from build123d import *

# Parameters (mm, degrees)
SKETCH1_W                                            = 380
SKETCH1_H                                            = 68
BOSS_EXTRUDE1_DEPTH                                  = 25
SKETCH2_R                                            = 28.5
CUT_EXTRUDE1_DEPTH                                   = 195.630419
CUT_EXTRUDE2_DEPTH                                   = 195.630419
CUT_EXTRUDE2_DEPTH_BACK                              = 195.630419
SKETCH4_R                                            = 9.55
CHAMFER1_SIZE                                        = 0.5
FILLET1_R                                            = 12
M8_CLEARANCE_HOLE1_D                                 = 9
CHAMFER2_SIZE                                        = 0.5
CHAMFER3_SIZE                                        = 0.5
M6X1_0_TAPPED_HOLE1_D                                = 5
SKETCH13_R                                           = 13.411040831
SKETCH13_R_2                                         = 14.724493856
BOSS_EXTRUDE3_DEPTH                                  = 8
CSK_FOR_5_16_FLAT_HEAD_SOCKET_CAP_SCREW1_D           = 8.4328
CSK_FOR_5_16_FLAT_HEAD_SOCKET_CAP_SCREW1_CSINK_D     = 18.4009792
CSK_FOR_5_16_FLAT_HEAD_SOCKET_CAP_SCREW1_CSINK_ANGLE = 82


with BuildPart() as part:
    # Sketch1 → Boss-Extrude1 (new body)
    with BuildSketch(Plane(origin=(0, 0, 0), x_dir=(1, 0, 0), z_dir=(0, 1, 0))):
        Rectangle(SKETCH1_W, SKETCH1_H)
    extrude(amount=BOSS_EXTRUDE1_DEPTH)

    # Sketch2 → Cut-Extrude1 (cut, through all)
    with BuildSketch(Plane(origin=(0, 25, 0), x_dir=(1, 0, 0), z_dir=(0, 1, 0))):
        with Locations(Location((-134, 0, 0), (0, 0, 270))):
            Circle(SKETCH2_R)
        with Locations(Location((134, 0, 0), (0, 0, 270))):
            Circle(SKETCH2_R)
    extrude(amount=-CUT_EXTRUDE1_DEPTH, mode=Mode.SUBTRACT)

    # Sketch4 → Cut-Extrude2 (cut, two sides: drawn at the far end of the back side and taken through both)
    with BuildSketch(Plane(origin=(0, 25, 0), x_dir=(1, 0, 0), z_dir=(0, 1, 0)).offset(-CUT_EXTRUDE2_DEPTH_BACK)):
        with Locations(Location((-46, 0, 0), (0, 0, 270))):
            Circle(SKETCH4_R)
        with Locations(Location((46, 0, 0), (0, 0, 270))):
            Circle(SKETCH4_R)
    extrude(amount=CUT_EXTRUDE2_DEPTH + CUT_EXTRUDE2_DEPTH_BACK, mode=Mode.SUBTRACT)

    # Chamfer1
    chamfer1_edges = [part.edges().sort_by_distance(p)[0] for p in [
        (-134, 0, -28.5),
        (-134, 25, -28.5),
        (134, 0, -28.5),
        (134, 25, -28.5),
        (-46, 0, -9.55),
        (-46, 25, -9.55),
        (46, 0, -9.55),
        (46, 25, -9.55),
    ]]
    chamfer(chamfer1_edges, length=CHAMFER1_SIZE)

    # Fillet1
    fillet1_edges = [part.edges().sort_by_distance(p)[0] for p in [
        (190, 12.5, 34),
        (-190, 12.5, 34),
        (-190, 12.5, -34),
        (190, 12.5, -34),
    ]]
    fillet(fillet1_edges, radius=FILLET1_R)

    # M8 Clearance Hole1 (through all)
    with Locations(Plane.XZ):
        with Locations((-178, -22), (-178, 22), (178, -22), (178, 22)):
            Hole(M8_CLEARANCE_HOLE1_D / 2)

    # Chamfer2
    chamfer2_edges = [part.edges().sort_by_distance(p)[0] for p in [
        (190, 0, 0),
        (0, 0, 34),
        (-190, 0, 0),
        (0, 0, -34),
        (-186.485281374, 0, 30.485281374),
        (-186.485281374, 0, -30.485281374),
        (186.485281374, 0, -30.485281374),
        (186.485281374, 0, 30.485281374),
    ]]
    chamfer(chamfer2_edges, length=CHAMFER2_SIZE)

    # Chamfer3
    chamfer3_edges = [part.edges().sort_by_distance(p)[0] for p in [
        (-173.5, 0, 22),
        (-173.5, 25, 22),
        (-173.5, 0, -22),
        (-173.5, 25, -22),
        (190, 25, 0),
        (0, 25, 34),
        (0, 25, -34),
        (-190, 25, 0),
        (-186.485281374, 25, 30.485281374),
        (-186.485281374, 25, -30.485281374),
        (186.485281374, 25, -30.485281374),
        (186.485281374, 25, 30.485281374),
        (182.5, 0, 22),
        (182.5, 25, 22),
        (182.5, 0, -22),
        (182.5, 25, -22),
    ]]
    chamfer(chamfer3_edges, length=CHAMFER3_SIZE)

    # M6x1.0 Tapped Hole1 (through all)
    with Locations(Plane(origin=(0, 0, 0), x_dir=(-1, 0, 0), z_dir=(0, -1, 0))):
        with Locations((158.765, -24.765), (109.235, -24.765), (109.235, 24.765), (158.765, 24.765), (-109.235, -24.765), (-158.765, -24.765), (-109.235, 24.765), (-158.765, 24.765)):
            Hole(M6X1_0_TAPPED_HOLE1_D / 2)

    # Sketch13 → Boss-Extrude3 (add)
    with BuildSketch(Plane(origin=(0, 25, 0), x_dir=(1, 0, 0), z_dir=(0, 1, 0))):
        with Locations((46, 0)):
            Circle(SKETCH13_R)
        with Locations((-46, 0)):
            Circle(SKETCH13_R_2)
    extrude(amount=-BOSS_EXTRUDE3_DEPTH)

    # CSK for 5/16 Flat Head Socket Cap Screw1 (through all)
    with Locations(Plane(origin=(0, 25, 0), x_dir=(1, 0, 0), z_dir=(0, 1, 0))):
        with Locations((46, 0), (-46, 0)):
            CounterSinkHole(CSK_FOR_5_16_FLAT_HEAD_SOCKET_CAP_SCREW1_D / 2, CSK_FOR_5_16_FLAT_HEAD_SOCKET_CAP_SCREW1_CSINK_D / 2, counter_sink_angle=CSK_FOR_5_16_FLAT_HEAD_SOCKET_CAP_SCREW1_CSINK_ANGLE)


solid = part.part
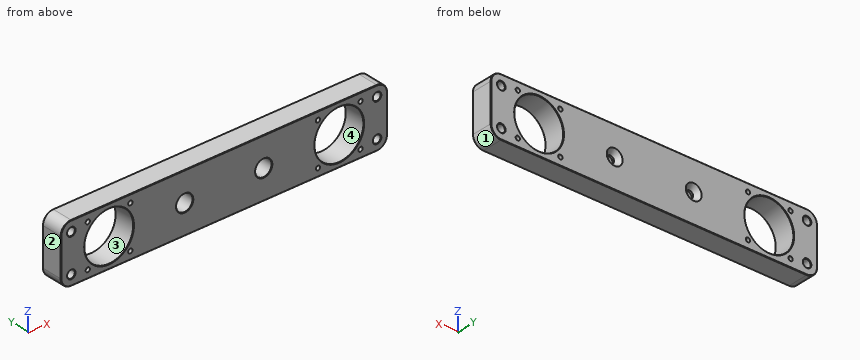
Input: part model. Units: mm. Frame: model coordinates. Face numbers are marked on the shaded views. Coordinates: 2 decimals unless noted, no trailing zeros. Loops run counter-clockwise (first coordinate to the right, second up) from the corner with the lowest first, then second, coordinate; pieces in that order, holes last.
(1) Pull-direction query (Z, two-part tool) for the marked faces 1, 2, 3 and 4; classes: released by +Z, released by -Z, zero draft, split by the parting line, or undercut.
(2) First-contact query: pin 1 Ø9.5 at (x, z) = (46, 0) entering from -Y. Flat tip, straight axial feed; report the tip coordinate or a pass-through.
(3) Section D-D on x = 134. Return the cut outline in (y, z), then the cut area to 3 significant figures.
(4) Material intervals for probe 1 along X at (y, z) = (20.5, 12.5); probe 2 along X at (y, z) = (21.5, -11.5); probe 3 along Z at (x, y) = (178, 8.25), sorted ascending.
(5) Section A-A on x = 46. Return the cut outline in (y, z).
(6) Section B-B on y = 7.5. Count the separate pieces of the cut face and the enclosed holes in it, then the cut area to 3 significant figures.
Data:
1. face 1: released by -Z
1. face 2: zero draft
1. face 3: undercut
1. face 4: undercut
2. pin 1: stops at y = 17
3. outline: (0, -33.5) - (0.5, -34) - (24.5, -34) - (25, -33.5) - (25, -29) - (24.5, -28.5) - (0.5, -28.5) - (0, -29) - close; (0, 29) - (0.5, 28.5) - (24.5, 28.5) - (25, 29) - (25, 33.5) - (24.5, 34) - (0.5, 34) - (0, 33.5) - close
3. area: 274 mm2
4. probe 1: x = -190 to -159.61, -108.39 to 108.39, 159.61 to 190
4. probe 2: x = -190 to -160.08, -107.92 to 107.92, 160.08 to 190
4. probe 3: z = -34 to -26.5, -17.5 to 17.5, 26.5 to 34
5. outline: (0, -33.5) - (0.5, -34) - (24.5, -34) - (25, -33.5) - (25, -9.2) - (19.27, -4.22) - (17, -4.22) - (17, -9.55) - (0.5, -9.55) - (0, -10.05) - close; (0, 10.05) - (0.5, 9.55) - (17, 9.55) - (17, 4.22) - (19.27, 4.22) - (25, 9.2) - (25, 33.5) - (24.5, 34) - (0.5, 34) - (0, 33.5) - close
6. separate pieces: 1
6. enclosed holes: 16
6. area: 19,600 mm2
